```python
from build123d import *

# Parameters (mm, degrees)
EXTRUDE_1_DEPTH = 27.58
EXTRUDE_START   = -10
EXTRUDE_2_DEPTH = 10


with BuildPart() as part:
    # 草圖1 → 伸長-薄件1 (new body)
    with BuildSketch(Plane(origin=(0, 0, 0), x_dir=(1, 0, 0), z_dir=(0, 1, 0))):
        with BuildLine():
            ThreePointArc((0, 5.1), (-5.1, 0), (0, -5.1))
            Line((0, -5.1), (0, -10.3))
            ThreePointArc((0, -10.3), (-10.3, 0), (0, 10.3))
            Line((0, 10.3), (0, 5.1))
        make_face()
    extrude(amount=EXTRUDE_1_DEPTH)

    # 草圖3 → 伸長-薄件2 (add)
    with BuildSketch(Plane(origin=(0, 27.58, 0), x_dir=(1, 0, 0), z_dir=(0, 1, 0)).offset(EXTRUDE_START)):
        with BuildLine():
            ThreePointArc((0, -5.1), (5.1, 0), (0, 5.1))
            Line((0, 5.1), (0, 10.3))
            ThreePointArc((0, 10.3), (10.3, 0), (0, -10.3))
            Line((0, -10.3), (0, -5.1))
        make_face()
    extrude(amount=EXTRUDE_2_DEPTH)


solid = part.part
```
The listing builds one solid part. Answer for the finished solid, in the listing's coordinates (mm). A direction names the side the tool comes from. Give positions to 0.01 mm unless a question says otherwise; leave off trailing zeros. Order: outer loops, then holes, each group sorted by start corner. A loop starts at its lowest first (then second) coordinate and runs counter-clockwise, first axis right, second up.
1) For faces 1 (the face through (0, 9, -8)), 2 (the face through (5, 27.58, 2)), determine the directions among +Z, -Z, +X, -X, +Y, -Y from which every point of the face is accessible in a straight line to the end or side of a thin tool.
Reported:
face 1: +Z, -Z, +X, -Y
face 2: +Z, -Z, +X, -X, +Y
2) Consider line 1 along Y through (x, z) = (3.5, 4); line 2 along X through (y, z) = (15.75, 0); line 3 along X through (y, z) = (20.75, 3). Determine where each line is inside the solid, lowest interval first.
Reported:
line 1: y = 17.58 to 27.58
line 2: x = -10.3 to -5.1
line 3: x = -9.85 to -4.12, 4.12 to 9.85
3) Find section B-B on x = -1.75. Write down the section's boundary in (y, z).
Reported:
outline: (0, -10.15) - (27.58, -10.15) - (27.58, -4.79) - (0, -4.79) - close; (0, 4.79) - (27.58, 4.79) - (27.58, 10.15) - (0, 10.15) - close
4) Given P1, Ø6, axis at x = 6.5, z = 4, coming from the -Y side; P2, Ø1, axis at x = -7.5, y = 20.5, coming from the +Z side; P3, Ø12, axis at y = 10.5, z = 8, coming from the +X side, each flat-ended and moving along its own axis, determine where each tip first touches the part or whether it passes through.
Reported:
P1: stops at y = 17.58
P2: stops at z = 7.56
P3: stops at x = 0
5) Determine the mould class of faces 3 (the face through (-9.14, 16.66, -4.75)), 4 (the face through (-4.5, 16.7, 2.4)), 5 (the face through (6, 17.58, 0)), 6 (the face through (0, 9, 8)) for opening direction X: pulls with the +X half, pulls with the -X half, needs draft (parallel to the pull), parting line crosses it, or undercut.
Reported:
face 3: parting line crosses it
face 4: undercut
face 5: needs draft
face 6: pulls with the +X half
6) Find section A-A on z = 0. Write down the section's boundary in (x, y), then the cut area to 3 significant figures.
Reported:
outline: (-10.3, 0) - (-5.1, 0) - (-5.1, 27.58) - (-10.3, 27.58) - close; (5.1, 17.58) - (10.3, 17.58) - (10.3, 27.58) - (5.1, 27.58) - close
area: 195 mm2
7) Find section D-D on y = 9.5. Write down the section's boundary in (x, z).
Reported:
outline: (0, -10.3) - (0, -5.1) arc R5.1 cw to (0, 5.1) - (0, 10.3) arc R10.3 ccw to start
8) Find section C-C on y = 23.75. Write down the section's boundary in (x, z).
Reported:
outline: circle Ø20.6 at (0, 0); hole circle Ø10.2 at (0, 0)
